from build123d import *

# Parameters (mm, degrees)
SKETCH1_W           = 10
SKETCH1_H           = 3
SKETCH1_W_2         = 3
BOSS_EXTRUDE1_DEPTH = 3


with BuildPart() as part:
    # Sketch1 → Boss-Extrude1 (new body)
    with BuildSketch(Plane.XY):
        Polygon((4.993890114, 24.809336695), (-61.106109886, 24.809336695), (-61.106109886, 13.809336695), (-58.106109886, 13.809336695), (-58.106109886, 3.809336695), (-61.106109886, 3.809336695), (-61.106109886, -13.190663305), (4.993890114, -13.190663305), (4.993890114, 3.809336695), (1.993890114, 3.809336695), (1.993890114, 13.809336695), (4.993890114, 13.809336695), align=None)
        with Locations((-28.056109886, -8.690663305)):
            Rectangle(SKETCH1_W, SKETCH1_H, mode=Mode.SUBTRACT)
        with Locations((-28.056109886, 20.309336695)):
            Rectangle(SKETCH1_W_2, SKETCH1_H, mode=Mode.SUBTRACT)
        with Locations((-8.056109886, -8.690663305)):
            Rectangle(SKETCH1_W, SKETCH1_H, mode=Mode.SUBTRACT)
        with Locations((-48.056109886, -8.690663305)):
            Rectangle(SKETCH1_W, SKETCH1_H, mode=Mode.SUBTRACT)
    extrude(amount=BOSS_EXTRUDE1_DEPTH)


solid = part.part
The model under review builds one solid part; all positions refer to its coordinate system, in mm. A direction names the side the tool comes from. Round coordinates to 2 decimals unless told otherwise and drop trailing zeros. Write each loop counter-clockwise with the first axis right and the second up, starting at its lowest first coordinate (ties: lowest second). Pieces come first, ordered by that corner, then holes. Notation, with made-up numbers: (40.5, -7) -> (99.5, -7) arc R14 cw to (99.5, 6) -> close; hole circle Ø11 at (38.25, 9.5). An arc over 180 degrees is marked (long way). Answer as a JSON object with one key per item and string values.
1. Clearance check with flat-ended pins moving along their axes: pin 1 (1.5 mm diameter, centred on x = -38, y = -4, fed in from -Z); pin 2 (1.5 mm diameter, centred on y = 11, z = 1, fed in from +X). State where each tip first meets the part, or that it passes through.
Results found:
{"pin 1": "stops at z = 0", "pin 2": "stops at x = 1.99"}
2. We need section D-D on z = 2.15. State the section outline as (x, y) points, and give its area (3 significant figures).
Results found:
{"outline": "(-61.11, -13.19) -> (4.99, -13.19) -> (4.99, 3.81) -> (1.99, 3.81) -> (1.99, 13.81) -> (4.99, 13.81) -> (4.99, 24.81) -> (-61.11, 24.81) -> (-61.11, 13.81) -> (-58.11, 13.81) -> (-58.11, 3.81) -> (-61.11, 3.81) -> close; hole (-53.06, -10.19) -> (-43.06, -10.19) -> (-43.06, -7.19) -> (-53.06, -7.19) -> close; hole (-33.06, -10.19) -> (-23.06, -10.19) -> (-23.06, -7.19) -> (-33.06, -7.19) -> close; hole (-29.56, 18.81) -> (-26.56, 18.81) -> (-26.56, 21.81) -> (-29.56, 21.81) -> close; hole (-13.06, -10.19) -> (-3.06, -10.19) -> (-3.06, -7.19) -> (-13.06, -7.19) -> close", "area": "2,350 mm^2"}
3. To check wall thickness, follow line 1 along X through (y, z) = (21.5, 1.2); line 2 along X through (y, z) = (4, 1.3); line 3 along Y through (x, z) = (-52.5, 1.4). State the ranges of each line that lie inside material, in increasing order.
Results found:
{"line 1": "x = -61.11 to -29.56, -26.56 to 4.99", "line 2": "x = -58.11 to 1.99", "line 3": "y = -13.19 to -10.19, -7.19 to 24.81"}
4. We need section A-A on y = -9. State the section outline as (x, z) points.
Results found:
{"outline": "(-61.11, 0) -> (-53.06, 0) -> (-53.06, 3) -> (-61.11, 3) -> close; (-43.06, 0) -> (-33.06, 0) -> (-33.06, 3) -> (-43.06, 3) -> close; (-23.06, 0) -> (-13.06, 0) -> (-13.06, 3) -> (-23.06, 3) -> close; (-3.06, 0) -> (4.99, 0) -> (4.99, 3) -> (-3.06, 3) -> close"}
5. The part is to be moulded in two halves that separate along Y. For faces 1 (the face through (-29, 6, 0)), 2 (the face through (-60, 3.809, 1)), 3 (the face through (-29, -13.191, 1)), say which applies: pulls with the +Y half, pulls with the -Y half, needs draft (parallel to the pull), parting line crosses it, or undercut.
Results found:
{"face 1": "needs draft", "face 2": "undercut", "face 3": "pulls with the -Y half"}
6. Machinability: for faces 4 (the face through (-60, 13.809, 1)), 5 (the face through (-8, -7.191, 1)), 6 (the face through (4, 3.809, 1)), 7 (the face through (4.994, 19, 1)), which of the approach directions +Z, -Z, +X, -X, +Y, -Y give a long, thin tool a straight path to every point of the face, cutting with its end or side? Answer none if there is none.
Results found:
{"face 4": "+Z, -Z, -X", "face 5": "+Z, -Z", "face 6": "+Z, -Z, +X", "face 7": "+Z, -Z, +X, +Y, -Y"}
7. We need section B-B on x = -4.5. State the section outline as (y, z) points.
Results found:
{"outline": "(-13.19, 0) -> (-10.19, 0) -> (-10.19, 3) -> (-13.19, 3) -> close; (-7.19, 0) -> (24.81, 0) -> (24.81, 3) -> (-7.19, 3) -> close"}
8. We need section C-C on y = 20. State the section outline as (x, z) points, and give its area (3 significant figures).
Results found:
{"outline": "(-61.11, 0) -> (-29.56, 0) -> (-29.56, 3) -> (-61.11, 3) -> close; (-26.56, 0) -> (4.99, 0) -> (4.99, 3) -> (-26.56, 3) -> close", "area": "189 mm^2"}
